from build123d import *

# Parameters (mm, degrees)
SKETCH_1_R      = 45
EXTRUDE_1_DEPTH = 40
FILLET_1_R      = 10


with BuildPart() as part:
    # 草图1 → 凸台-拉伸1 (new body)
    with BuildSketch(Plane(origin=(0, 0, 0), x_dir=(1, 0, 0), z_dir=(0, 1, 0))):
        with BuildLine():
            Line((110, 0), (-110, 0))
            Line((-110, 0), (-110, 30))
            Line((-110, 30), (-90, 30))
            Line((-90, 30), (-72.360679775, 94.72135955))
            ThreePointArc((-72.360679775, 94.72135955), (0, 150), (72.360679775, 94.72135955))
            Line((72.360679775, 94.72135955), (90, 30))
            Line((90, 30), (110, 30))
            Line((110, 30), (110, 0))
        make_face()
        with Locations(Location((0, 75, 0), (0, 0, 270))):
            Circle(SKETCH_1_R, mode=Mode.SUBTRACT)
    extrude(amount=EXTRUDE_1_DEPTH)

    # 圆角1
    fillet_1_edges = [part.edges().sort_by_distance(p)[0] for p in [
        (-90, 20, -30),
        (90, 20, -30),
    ]]
    fillet(fillet_1_edges, radius=FILLET_1_R)


solid = part.part
Check sheet for the modelled part. Datum: model origin and axes. Units: mm. A direction names the side the tool comes from. Give positions to 0.01 mm unless a question says otherwise; leave off trailing zeros. Loops run counter-clockwise (first coordinate to the right, second up) from the corner with the lowest first, then second, coordinate; pieces in that order, holes last. Notation, with made-up numbers: M 17.25,-4.5 L 73.25,-4.5 A15 ccw 73.25,15.5 Z; hole C 0,-37.5 d2. An arc over 180 degrees is marked long. Answer as a JSON object with one key per item and string values. Group by question number.
Q1. Material ranges on line 1 along X through (y, z) = (15, -75); line 2 along X through (y, z) = (17, -101); line 3 along Z through (x, y) = (99.5, 32), recorded low to high. Write a range as [from, to].
Q2. Cross-section at D-D on x = 55. Record the cut outline in (y, z).
Q3. Go/stop test with flat-tipped pins: P1, Ø6, axis at y = 22.5, z = -51, coming from the -X side; P2, Ø3, axis at y = 25.5, z = -57.5, coming from the -X side; P3, Ø10, axis at x = 101.5, y = 13.5, coming from the -Z side. Record where each tip stops, or that it passes through.
Q4. Cross-section at C-C on z = -75. Record the cut outline in (x, y), then the cut area to 3 significant figures.
Q5. Access from +Z, -Z, +X, -X, +Y, -Y to the whole of each face (thin tool, end or side, straight path). Record for faces 5 (the flat face through (-104, 20, -30)), 6 (the flat face through (-110, 20, -15)), 7 (the flat face through (104, 20, -30)).
Q6. Cross-section at B-B on y = 28.5. Record the cut outline in (x, z), then the cut area to 3 significant figures.
Q7. Release check for a two-part mould opening along X. For faces 1 (the cylindrical face through (1.979, 19.72, -119.956)), 2 (the flat face through (2, 20, 0)), 3 (the cylindrical face through (-1.37, 19.72, -149.987)), 4 (the flat face through (110, 20, -15)) record: released by +X, released by -X, zero draft, split by the parting line, or undercut.
Q8. Cross-section at A-A on x = 0. Record the cut outline in (y, z).
Evaluation:
{
 "1": {"line 1": "x = [-77.74, -45], [45, 77.74]", "line 2": "x = [-70.35, -36.73], [36.73, 70.35]", "line 3": "z = [-30, 0]"},
 "2": {"outline": "M 0,-125.99 L 40,-125.99 L 40,0 L 0,0 Z"},
 "3": {"P1": "stops at x = -85.09", "P2": "stops at x = -82.91", "P3": "stops at z = -30.07"},
 "4": {"outline": "M -77.74,0 L -45,0 L -45,40 L -77.74,40 Z; M 45,0 L 77.74,0 L 77.74,40 L 45,40 Z", "area": "2,620 mm2"},
 "5": {"face 5": "-Z, -X, +Y, -Y", "face 6": "+Z, -Z, -X, +Y, -Y", "face 7": "-Z, +X, +Y, -Y"},
 "6": {"outline": "M -110,-30 L -97.64,-30 A10 cw -87.99,-37.37 L -72.36,-94.72 A75 ccw 72.36,-94.72 L 87.99,-37.37 A10 cw 97.64,-30 L 110,-30 L 110,0 L -110,0 Z; hole C 0,-75 d90", "area": "16,700 mm2"},
 "7": {"face 1": "undercut", "face 2": "zero draft", "face 3": "split by the parting line", "face 4": "released by +X"},
 "8": {"outline": "M 0,-150 L 40,-150 L 40,-120 L 0,-120 Z; M 0,-30 L 40,-30 L 40,0 L 0,0 Z"}
}
